```python
from build123d import *

# Parameters (mm, degrees)
F0_R     = 15
F0_R_2   = 10
F1_DEPTH = 10


# Not quite as in the source:
# - a feature names something its author has since deleted; it is built from what else it names


with BuildPart() as f1:
    # F0 (on Top) → F1 (new body)
    with BuildSketch(Plane.XY):
        with BuildLine():
            ThreePointArc((42.0721931458, -20.106328072), (15.2726376348, 3.6807596445), (8.0721931458, 38.7833993854))
            ThreePointArc((8.0721931458, 38.7833993854), (9.5591074328, 40.6079882936), (11.8827049224, 40.9833993854))
            ThreePointArc((11.8827049224, 40.9833993854), (12.6879608107, 43.9886552737), (9.6827049224, 44.793911162))
            ThreePointArc((9.6827049224, 44.793911162), (8.1957906353, 42.9693222537), (5.8721931458, 42.593911162))
            ThreePointArc((5.8721931458, 42.593911162), (0, 44.17956576), (-5.8721931458, 42.593911162))
            ThreePointArc((-5.8721931458, 42.593911162), (-8.1957906353, 42.9693222537), (-9.6827049224, 44.793911162))
            ThreePointArc((-9.6827049224, 44.793911162), (-12.6879608107, 43.9886552737), (-11.8827049224, 40.9833993854))
            ThreePointArc((-11.8827049224, 40.9833993854), (-9.5591074328, 40.6079882936), (-8.0721931458, 38.7833993854))
            ThreePointArc((-8.0721931458, 38.7833993854), (-15.2726376348, 3.6807596445), (-42.0721931458, -20.106328072))
            ThreePointArc((-42.0721931458, -20.106328072), (-44.3957906353, -19.7309169803), (-45.8827049224, -17.906328072))
            ThreePointArc((-45.8827049224, -17.906328072), (-48.8879608107, -18.7115839603), (-48.0827049224, -21.7168398486))
            ThreePointArc((-48.0827049224, -21.7168398486), (-45.7591074328, -22.0922509404), (-44.2721931458, -23.9168398486))
            ThreePointArc((-44.2721931458, -23.9168398486), (-42.7651143596, -28.4458898793), (-38.4, -30.3770442686))
            ThreePointArc((-38.4, -30.3770442686), (-37.5391516656, -32.6039224965), (-38.4, -34.8308007245))
            ThreePointArc((-38.4, -34.8308007245), (-36.2, -37.010864664), (-34, -34.8308007245))
            ThreePointArc((-34, -34.8308007245), (-34.8608483344, -32.6039224965), (-34, -30.3770442686))
            ThreePointArc((-34, -30.3770442686), (0, -15.1188267986), (34, -30.3770442686))
            ThreePointArc((34, -30.3770442686), (34.8608483344, -32.6039224965), (34, -34.8308007245))
            ThreePointArc((34, -34.8308007245), (36.2, -37.010864664), (38.4, -34.8308007245))
            ThreePointArc((38.4, -34.8308007245), (37.5391516656, -32.6039224965), (38.4, -30.3770442686))
            ThreePointArc((38.4, -30.3770442686), (42.7651143596, -28.4458898793), (44.2721931458, -23.9168398486))
            ThreePointArc((44.2721931458, -23.9168398486), (45.7591074328, -22.0922509404), (48.0827049224, -21.7168398486))
            ThreePointArc((48.0827049224, -21.7168398486), (48.8879608107, -18.7115839603), (45.8827049224, -17.906328072))
            ThreePointArc((45.8827049224, -17.906328072), (44.3957906353, -19.7309169803), (42.0721931458, -20.106328072))
        make_face()
        Circle(F0_R, mode=Mode.SUBTRACT)
        Circle(F0_R)
        Circle(F0_R_2, mode=Mode.SUBTRACT)
    extrude(amount=F1_DEPTH)


solid = f1.part
```
Geometry: final body of the model. Coordinates: model frame, mm. A direction names the side the tool comes from. Coordinates: 2 decimals unless noted, no trailing zeros. Loops run counter-clockwise (first coordinate to the right, second up) from the corner with the lowest first, then second, coordinate; pieces in that order, holes last. Notation, with made-up numbers: (70.25, -0.75) -> (122.25, -0.75) arc R23 ccw to (122.25, 23.25) -> close; hole circle Ø7 at (-34, 33.25). An arc over 180 degrees is marked (long way). Use a Markdown table: item, result. Add a question column.
(1) Section query C-C, the plane y = -3. Return loops of the section in (x, z).
(2) Section query D-D, the plane y = 29.5. Return loops of the section in (x, z), plus the area to 3 significant figures.
(3) Access query for faces 4 (the cylindrical face through (34.86, -32.57, 4.93)), 5 (the cylindrical face through (44.425, -19.714, 4.93)). Directions: +Z, -Z, +X, -X, +Y, -Y. A direction counts if a zero-diameter tool reaches every point of the face in a straight line with its end or side. Return the directions, or none.
(4) Mould query, pull axis Y, two halves, no side actions, for faces 1 (the cylindrical face through (0.09, 44.18, 4.93)), 2 (the cylindrical face through (-36, -37, 5)), 3 (the cylindrical face through (-15.02, 4.12, 4.93)). Classes: pulls with the +Y half, pulls with the -Y half, needs draft (parallel to the pull), parting line crosses it, or undercut.
(5) Line query: line 1 along Y through (x, z) = (0, 7.5); line 2 along Y through (x, z) = (7, 7.25); line 3 along X through (y, z) = (-18.5, 1.75). Output: solid intervals per line, ascending.
(6) Pin query (flat end, axial travel): pin 1 Ø1.5 at (x, z) = (5, 8) entering from +Y; pin 2 Ø5 at (y, z) = (34, 3.5) entering from -X; pin 3 Ø5 at (y, z) = (9.5, 2.5) entering from -X; pin 4 Ø1.5 at (x, y) = (10, 31.5) entering from +Z. Return the tip coordinate at first contact, or that it passes through.
(7) Section query B-B, the plane z = 3.75. Return loops of the section in (x, y), plus the area to 3 significant figures.
(8) Section query A-A, the plane x = 0. Return loops of the section in (y, z).
Answer:
| question | item | result |
|---|---|---|
| 1 | outline | (-19.79, 0) -> (-9.54, 0) -> (-9.54, 10) -> (-19.79, 10) -> close; (9.54, 0) -> (19.79, 0) -> (19.79, 10) -> (9.54, 10) -> close |
| 2 | outline | (-7.73, 0) -> (7.73, 0) -> (7.73, 10) -> (-7.73, 10) -> close |
| 2 | area | 155 mm^2 |
| 3 | face 4 | +Z, -Z |
| 3 | face 5 | +Z, -Z, +Y |
| 4 | face 1 | pulls with the +Y half |
| 4 | face 2 | pulls with the -Y half |
| 4 | face 3 | undercut |
| 5 | line 1 | y = -15.12 to -10, 10 to 44.18 |
| 5 | line 2 | y = -15.66 to -7.14, 7.14 to 42.56 |
| 5 | line 3 | x = -48.75 to -45.62, -38.64 to -17.21, 17.21 to 38.64, 45.62 to 48.75 |
| 6 | pin 1 | stops at y = 43.38 |
| 6 | pin 2 | stops at x = -7.85 |
| 6 | pin 3 | stops at x = -13.5 |
| 6 | pin 4 | passes through |
| 7 | outline | (-48.08, -21.72) arc R3.31 cw to (-44.27, -23.92) arc R5.9 ccw to (-38.4, -30.38) arc R3.31 cw to (-38.4, -34.83) arc R2.2 ccw to (-34, -34.83) arc R3.31 cw to (-34, -30.38) arc R45.51 cw to (34, -30.38) arc R3.31 cw to (34, -34.83) arc R2.2 ccw to (38.4, -34.83) arc R3.31 cw to (38.4, -30.38) arc R5.9 ccw to (44.27, -23.92) arc R3.31 cw to (48.08, -21.72) arc R2.2 ccw to (45.88, -17.91) arc R3.31 cw to (42.07, -20.11) arc R56.74 cw to (8.07, 38.78) arc R3.31 cw to (11.88, 40.98) arc R2.2 ccw to (9.68, 44.79) arc R3.31 cw to (5.87, 42.59) arc R11.67 ccw to (-5.87, 42.59) arc R3.31 cw to (-9.68, 44.79) arc R2.2 ccw to (-11.88, 40.98) arc R3.31 cw to (-8.07, 38.78) arc R56.74 cw to (-42.07, -20.11) arc R3.31 cw to (-45.88, -17.91) arc R2.2 ccw to start; hole circle Ø20 at (0, 0) |
| 7 | area | 1,960 mm^2 |
| 8 | outline | (-15.12, 0) -> (-10, 0) -> (-10, 10) -> (-15.12, 10) -> close; (10, 0) -> (44.18, 0) -> (44.18, 10) -> (10, 10) -> close |
